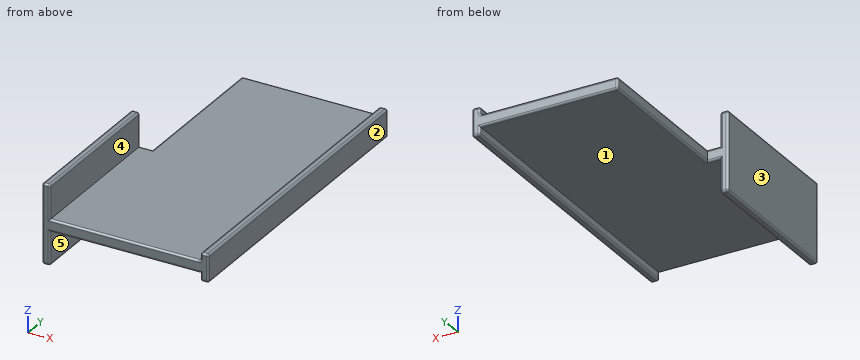
Autodesk Inventor part; units mm, degrees
ref_plane "YZ Plane" through (0, 0, 0) normal (1, 0, 0) x (0, 1, 0)
ref_plane "XZ Plane" through (0, 0, 0) normal (0, 1, 0) x (-1, 0, 0)
ref_plane "XY Plane" through (0, 0, 0) normal (0, 0, 1) x (1, 0, 0)
sketch "スケッチ1" plane through (0, 0, 0) normal (0, 1, 0) x (-1, 0, 0)
  line L0 (0, 0) -> (-40, 0)
  line L1 (-40, 0) -> (-40, -3)
  line L2 (-40, -3) -> (0, -3)
  line L3 (0, -3) -> (0, 0)
  line L4 (-39, 2) -> (-41, 2)
  line L5 (-41, 2) -> (-41, -5)
  line L6 (-41, -5) -> (-39, -5)
  line L7 (-39, -5) -> (-39, 2)
  line L8 (-39, 2) -> (-41, -5) construction
  line L9 (-41, 2) -> (-39, -5) construction
  line L10 (1, 8.5) -> (-1, 8.5)
  line L11 (-1, 8.5) -> (-1, -11.5)
  line L12 (-1, -11.5) -> (1, -11.5)
  line L13 (1, -11.5) -> (1, 8.5)
  line L14 (1, 8.5) -> (-1, -11.5) construction
  line L15 (-1, 8.5) -> (1, -11.5) construction
  point P0 (-40, -1.5)
  point P1 (0, -1.5)
  dimension "d1" = 40
  dimension "d2" = 3
  dimension "d3" = 2
  dimension "d4" = 7
  dimension "d5" = 2
  dimension "d6" = 20
extrude "押し出し1" add sketch "スケッチ1" along normal blind 78
sketch "スケッチ2" plane through (0, 78, 0) normal (0, 1, 0) x (1, 0, 0)
  line L0 (1, 3) -> (1, 11.5)
  line L1 (-1, -8.5) -> (1, -8.5)
  line L2 (1, -8.5) -> (1, 11.5)
  line L3 (1, 11.5) -> (-1, 11.5)
  line L4 (-1, 11.5) -> (-1, -8.5)
  line L5 (1, 0) -> (39, 0)
  line L6 (1, 0) -> (4.2, 0)
  line L7 (4.2, 0) -> (4.2, 3)
  line L8 (4.2, 3) -> (1, 3)
  line L9 (1, 3) -> (1, 0)
  point P0 (0, 0)
  dimension "d9" = 2
  dimension "d10" = 20
  dimension "d11" = 3.2
  dimension "d12" = 3
extrude "押し出し2" cut sketch "スケッチ2" against normal blind 39
fillet "フィレット1" radius 0.5 38 edges at (1, 0, 4.25) (-1, 0, -1.5) (1, 19.5, 8.5) (0, 0, -11.5) (1, 0, -7.25) (20, 0, 0) (20, 0, -3) (0, 0, 8.5) (41, 0, -1.5) (40, 0, 2) (39, 39, 0) (40, 0, -5) (39, 0, 1) (39, 0, -4) (41, 39, -5) (39, 39, -5) (41, 39, 2) (41, 78, -1.5) (40, 78, -5) (21.6, 78, -3) (4.2, 58.5, 0) (2.6, 39, 0) (1, 39, 4.25) (0, 39, 8.5) (-1, 19.5, 8.5) (39, 39, 2) (21.6, 78, 0) (40, 78, 2) (39, 78, 1) (4.2, 78, -1.5) (4.2, 58.5, -3) (39, 78, -4) (-1, 19.5, -11.5) (1, 19.5, -11.5) (0, 39, -11.5) (1, 39, -7.25) (-1, 39, -1.5) (2.6, 39, -3)
properties part number "halfPartition"
CAD build for the part. Positions are in the model's coordinates, mm. Face numbers are marked on the shaded views. A direction names the side the tool comes from. Coordinates: 2 decimals unless noted, no trailing zeros. Loops run counter-clockwise (first coordinate to the right, second up) from the corner with the lowest first, then second, coordinate; pieces in that order, holes last. Notation, with made-up numbers: (72.5, 66) - (92.5, 66) arc R10 ccw to (92.5, 72) - close; hole circle Ø3 at (10.25, 6.5). An arc over 180 degrees is marked (long way). Return JSON: item names as keys, results as strings.
1. Mould opens along X. For the marked faces 1, 2 and 3 say: released by +X, released by -X, zero draft, split by the parting line, or undercut.
Result:
{"face 1": "undercut", "face 2": "released by +X", "face 3": "released by -X"}
2. Drop flat-ended pins along their axis: pin 1 (6.5 mm diameter, centred on y = 24.5, z = 5, fed in from +X); pin 2 (1.4 mm diameter, centred on x = 1.5, z = -4.5, fed in from +Y); pin 3 (1.6 mm diameter, centred on y = 62, z = -1.5, fed in from -X). Give the stop position or say it passes through.
Result:
{"pin 1": "stops at x = 40.93", "pin 2": "stops at y = 38.9", "pin 3": "stops at x = 4.2"}
3. Band-saw the part on D-D (y = 60). Give the cut face in (x, z), and give its area (3 significant figures).
Result:
{"outline": "(4.2, -2.5) arc R0.5 ccw to (4.7, -3) - (39, -3) - (39, -4.5) arc R0.5 ccw to (39.5, -5) - (40.5, -5) arc R0.5 ccw to (41, -4.5) - (41, 1.5) arc R0.5 ccw to (40.5, 2) - (39.5, 2) arc R0.5 ccw to (39, 1.5) - (39, 0.5) arc R0.5 cw to (38.5, 0) - (4.7, 0) arc R0.5 ccw to (4.2, -0.5) - close", "area": "118 mm2"}
4. Probe L1, parallel to X at y = 34.5, z = 0.75; L2, parallel to Z at x = 28, y = 21; L3, parallel to X at y = 46.5, z = -1.25. List the from-to ranges inside material, lowest first. Write a range as from..to.
Result:
{"L1": "x = -1..1, 39..41", "L2": "z = -3..0", "L3": "x = 4.2..41"}
5. 3-axis set-ups, long thin cutter, end or side, ignore diameter. For the marked faces 4 and 5: which of +Z, -Z, +X, -X, +Y, -Y reach the whole face in a straight line?
Result:
{"face 4": "+Z, +Y, -Y", "face 5": "-Z, +Y, -Y"}
6. Band-saw the part on C-C (x = 33.5). Give the cut face in (y, z), and give its area (3 significant figures).
Result:
{"outline": "(0, -2.5) arc R0.5 ccw to (0.5, -3) - (77.5, -3) arc R0.5 ccw to (78, -2.5) - (78, -0.5) arc R0.5 ccw to (77.5, 0) - (0.5, 0) arc R0.5 ccw to (0, -0.5) - close", "area": "234 mm2"}
7. Band-saw the part on B-B (y = 18.5). Give the cut face in (x, z), and give its area (3 significant figures).
Result:
{"outline": "(-1, -11) arc R0.5 ccw to (-0.5, -11.5) - (0.5, -11.5) arc R0.5 ccw to (1, -11) - (1, -3) - (39, -3) - (39, -4.5) arc R0.5 ccw to (39.5, -5) - (40.5, -5) arc R0.5 ccw to (41, -4.5) - (41, 1.5) arc R0.5 ccw to (40.5, 2) - (39.5, 2) arc R0.5 ccw to (39, 1.5) - (39, 0.5) arc R0.5 cw to (38.5, 0) - (1, 0) - (1, 8) arc R0.5 ccw to (0.5, 8.5) - (-0.5, 8.5) arc R0.5 ccw to (-1, 8) - close", "area": "168 mm2"}
8. Band-saw the part on A-A (z = 5.75). Give the cut face in (x, y).
Result:
{"outline": "(-1, 0.5) arc R0.5 ccw to (-0.5, 0) - (0.5, 0) arc R0.5 ccw to (1, 0.5) - (1, 38.5) arc R0.5 ccw to (0.5, 39) - (-0.5, 39) arc R0.5 ccw to (-1, 38.5) - close"}
